Input: part model. Units: mm. Frame: model coordinates. A direction names the side the tool comes from. Coordinates: 2 decimals unless noted, no trailing zeros. Loops run counter-clockwise (first coordinate to the right, second up) from the corner with the lowest first, then second, coordinate; pieces in that order, holes last. Notation, with made-up numbers: (89, 11.25) - (100, 11.25) arc R18 ccw to (100, 21.25) - close; hole circle Ø11 at (-20.75, 31). An arc over 180 degrees is marked (long way). Use one line per item in the form item = value.
from build123d import *

# Parameters (mm, degrees)
PAD025_DEPTH    = 53
SKETCH054_W     = 1.8
SKETCH054_H     = 1.8
POCKET026_DEPTH = 2
SKETCH119_W     = 2.4
SKETCH119_H     = 4.6
POCKET052_DEPTH = 0.2


with BuildPart() as part:
    # Sketch052 → Pad025 (new body)
    with BuildSketch(Plane.XZ):
        with BuildLine():
            ThreePointArc((-14.414866, 3.546381), (-17.164866, 0.796381), (-14.414866, -1.953619))
            Line((-14.414866, -1.953619), (14.085134, -1.953619))
            ThreePointArc((14.085134, -1.953619), (16.835134, 0.796381), (14.085134, 3.546381))
            Line((-14.414866, 3.546381), (14.085134, 3.546381))
        make_face()
    extrude(amount=PAD025_DEPTH)

    # Sketch054 (on Face2 of Pad025) → Pocket026 (cut)
    with BuildSketch(Plane(origin=(0, 0, -1.953619), x_dir=(1, 0, 0), z_dir=(0, 0, -1))):
        with Locations((-16.201848, 52.106387)):
            Rectangle(SKETCH054_W, SKETCH054_H)
        with Locations((15.881731, 52.106387)):
            Rectangle(SKETCH054_W, SKETCH054_H)
    extrude(amount=-POCKET026_DEPTH, mode=Mode.SUBTRACT)

    # Sketch119 (on Face4 of Pocket026) → Pocket052 (cut)
    with BuildSketch(Plane.XZ.offset(53)):
        with Locations((-12.97, 0.818601)):
            Rectangle(SKETCH119_W, SKETCH119_H)
        with Locations((-10.17, 0.818601)):
            Rectangle(SKETCH119_W, SKETCH119_H)
        with Locations((-7.37, 0.818601)):
            Rectangle(SKETCH119_W, SKETCH119_H)
    extrude(amount=-POCKET052_DEPTH, mode=Mode.SUBTRACT)


with BuildPart() as part_1:
    # Body007 placement: moved
    add(part.part.moved(Location((-0.6, 34, -4.5))))


solid = part_1.part
Q1. Pull-direction query (Z, two-part tool) for faces 6 (the flat face through (-17, -18, -4.454)), 7 (the flat face through (-1, -19, -4)), 8 (the flat face through (-11, -18.8, -4)), 9 (the flat face through (-8, -18.8, -4)); classes: pulls with the +Z half, pulls with the -Z half, needs draft (parallel to the pull), parting line crosses it, or undercut.
Check values:
face_6 = pulls with the -Z half
face_7 = needs draft
face_8 = undercut
face_9 = undercut
Q2. Set-up query: faces 1 (the cylindrical face through (-17.764, 7.871, -3.643)), 2 (the flat face through (-14, -18.8, -4)), 3 (the flat face through (14.382, -18, -5)), 4 (the flat face through (-1, 8, -6.454)), 5 (the flat face through (-15.902, -18, -5)). Return all of +Z, -Z, +X, -X, +Y, -Y with unobstructed straight access to the full face (end or side cutting, diameter ignored); none if empty.
Check values:
face_1 = -X, +Y, -Y
face_2 = -Y
face_3 = -Z, +X, -Y
face_4 = -Z, +X, -X, +Y, -Y
face_5 = -Z, -X, -Y
Q3. Ray query, line 1 along X through (y, z) = (24, -3.45); line 2 along Y through (x, z) = (-7.5, -3.45); line 3 along Y through (x, z) = (-16, -5.7). Return the intervals inside material, ascending. Write a range as [from, to].
Check values:
line_1 = [-17.75, 16.22]
line_2 = [-18.8, 34]
line_3 = [-17.21, 34]
Q4. Cut plane C-C, the plane z = -2.3. Return loops of the section in (x, y).
Check values:
outline = (-17.38, -19) - (-14.77, -19) - (-14.77, -18.8) - (-12.37, -18.8) - (-12.37, -19) - (-11.97, -19) - (-11.97, -18.8) - (-9.57, -18.8) - (-9.57, -19) - (-9.17, -19) - (-9.17, -18.8) - (-6.77, -18.8) - (-6.77, -19) - (15.85, -19) - (15.85, 34) - (-17.38, 34) - close
Q5. First-contact query: P1, Ø0.5, axis at y = -18.5, z = -5.5, coming from the +X side; P2, Ø3, axis at y = 9, z = -2, coming from the +X side; P3, Ø1.9, axis at x = 15.5, y = -18.5, coming from the -Z side. Flat tips, straight axial feed; report the tip coordinate or a pass-through.
Check values:
P1 = 14.38
P2 = 16.23
P3 = -4.45
Q6. Cut plane A-A, the plane z = -5.1. Return loops of the section in (x, y), then the cut area to 3 significant figures.
Check values:
outline = (-17.38, -17.21) - (-15.9, -17.21) - (-15.9, -19) - (-14.77, -19) - (-14.77, -18.8) - (-12.37, -18.8) - (-12.37, -19) - (-11.97, -19) - (-11.97, -18.8) - (-9.57, -18.8) - (-9.57, -19) - (-9.17, -19) - (-9.17, -18.8) - (-6.77, -18.8) - (-6.77, -19) - (14.38, -19) - (14.38, -17.21) - (15.85, -17.21) - (15.85, 34) - (-17.38, 34) - close
area = 1,750 mm²
Q7. Cut plane B-B, the plane y = 15. Return loops of the section in (x, z).
Check values:
outline = (-15.01, -6.45) - (13.49, -6.45) arc R2.75 ccw to (13.49, -0.95) - (-15.01, -0.95) arc R2.75 ccw to start
